Model file for the job. Use its own axes, mm. Face numbers are marked on the shaded views. Round coordinates to 2 decimals unless told otherwise and drop trailing zeros. Loops run counter-clockwise (first coordinate to the right, second up) from the corner with the lowest first, then second, coordinate; pieces in that order, holes last. Notation, with made-up numbers: (80, 49.25) -> (113, 49.25) arc R13 ccw to (113, 55.25) -> close; hole circle Ø10 at (-21.5, -27.75). An arc over 180 degrees is marked (long way). Use a Markdown table: item, result. Add a question column.
```python
from build123d import *

# Parameters (mm, degrees)
SKETCH1_R           = 5.175
SKETCH1_R_2         = 3.175
BOSS_EXTRUDE1_DEPTH = 5
SKETCH5_W           = 0.371171222
SKETCH5_H           = 5
CUT_EXTRUDE1_DEPTH  = 20
FILLET1_R           = 0.5


with BuildPart() as part:
    # Sketch1 → Boss-Extrude1 (new body)
    with BuildSketch(Plane.XY):
        Circle(SKETCH1_R)
        Circle(SKETCH1_R_2, mode=Mode.SUBTRACT)
    extrude(amount=BOSS_EXTRUDE1_DEPTH)

    # Sketch5 → Cut-Extrude1 (cut)
    with BuildSketch(Plane(origin=(0, 0, 0), x_dir=(1, 0, 0), z_dir=(0, 1, 0))):
        with Locations((0, -2.5)):
            Rectangle(SKETCH5_W, SKETCH5_H)
    extrude(amount=-CUT_EXTRUDE1_DEPTH, mode=Mode.SUBTRACT)

    # Fillet1
    fillet1_edges = [part.edges().sort_by_distance(p)[0] for p in [
        (0.185585611, -3.169571419, 2.5),
        (-0.185585611, -3.169571419, 2.5),
        (-0.185585611, -5.171671198, 2.5),
        (0.185585611, -5.171671198, 2.5),
    ]]
    fillet(fillet1_edges, radius=FILLET1_R)


solid = part.part
```
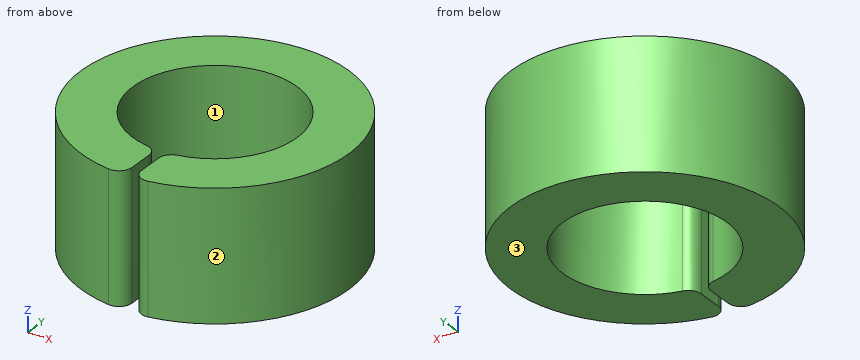
1) Wall check: probe 1 along X at (y, z) = (0, 2.8) (3 decimals); probe 2 along X at (y, z) = (-3.75, 2.2); probe 3 along Y at (x, z) = (1.5, 2). Give the ranges that are in metal, low to high. Write a range as from..to.
2) Cut at C-C on z = 0.45. Write the cut outline in (x, y) (3 decimals).
3) Cut at B-B on x = 2.75. Write the cut outline in (y, z).
4) Pin check, flat tips, straight feed: pin 1 Ø0.8 at (y, z) = (-4, 2) entering from -X; pin 2 Ø1.5 at (y, z) = (1.5, 2.5) entering from -X; pin 3 Ø1 at (x, z) = (-3.5, 3) entering from -Y. Stop position of each tip, or through.
5) Cut at A-A on y = 0. Write the cut outline in (x, z) (3 decimals).
6) Pull direction X, two halves, no side cores. Call the marked faces 1, 2 and 3: +X half, -X half, draft (parallel to the pull), parting line (faces both ways), or undercut.
7) Cut at D-D on x = 0. Write the cut outline in (y, z) (3 decimals).
Established:
| question | item | result |
|---|---|---|
| 1 | probe 1 | x = -5.175..-3.175, 3.175..5.175 |
| 1 | probe 2 | x = -3.57..-0.19, 0.19..3.57 |
| 1 | probe 3 | y = -4.95..-2.8, 2.8..4.95 |
| 2 | outline | (-0.759, -5.119) arc R0.5 ccw to (-0.186, -4.624) -> (-0.186, -3.61) arc R0.5 ccw to (-0.592, -3.119) arc R3.175 cw (long way) to (0.592, -3.119) arc R0.5 ccw to (0.186, -3.61) -> (0.186, -4.624) arc R0.5 ccw to (0.759, -5.119) arc R5.175 ccw (long way) to start |
| 3 | outline | (-4.38, 0) -> (-1.59, 0) -> (-1.59, 5) -> (-4.38, 5) -> close; (1.59, 0) -> (4.38, 0) -> (4.38, 5) -> (1.59, 5) -> close |
| 4 | pin 1 | stops at x = -3.72 |
| 4 | pin 2 | stops at x = -5.12 |
| 4 | pin 3 | stops at y = -4.22 |
| 5 | outline | (-5.175, 0) -> (-3.175, 0) -> (-3.175, 5) -> (-5.175, 5) -> close; (3.175, 0) -> (5.175, 0) -> (5.175, 5) -> (3.175, 5) -> close |
| 6 | face 1 | undercut |
| 6 | face 2 | parting line |
| 6 | face 3 | draft |
| 7 | outline | (3.175, 0) -> (5.175, 0) -> (5.175, 5) -> (3.175, 5) -> close |
